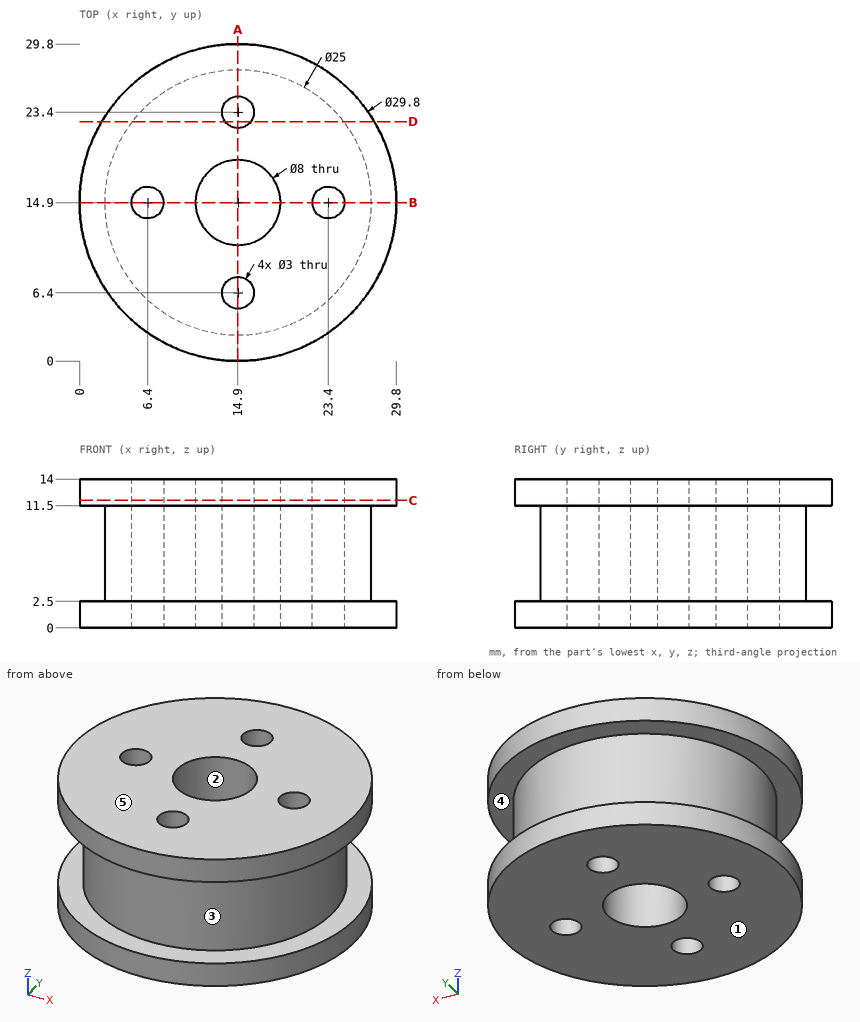
Geometry check sheet. Reference: drawing and pictorial views, mm from the part's lowest x, y, z. A direction names the side the tool comes from. Coordinates: 2 decimals unless noted, no trailing zeros. Order: outer loops, then holes, each group sorted by start corner. A loop starts at its lowest first (then second) coordinate and runs counter-clockwise, first axis right, second up. Notation, with made-up numbers: (-9, 70) - (18, 70) arc R20 cw to (18, 101) - close; hole circle Ø3 at (-20.75, -9.75). An arc over 180 degrees is marked (long way). One line per item, written item: value.
(1) Access from +Z, -Z, +X, -X, +Y, -Y to the whole of each face (thin tool, end or side, straight path). Record for the marked faces 4 and 5.
Data:
face 4: none
face 5: +Z, +X, -X, +Y, -Y
(2) Sectioned sample at A-A (x = 14.9). Enter the section's corners in (y, z).
Data:
outline: (0, 0) - (4.9, 0) - (4.9, 14) - (0, 14) - (0, 11.5) - (2.4, 11.5) - (2.4, 2.5) - (0, 2.5) - close; (7.9, 0) - (10.9, 0) - (10.9, 14) - (7.9, 14) - close; (18.9, 0) - (21.9, 0) - (21.9, 14) - (18.9, 14) - close; (24.9, 0) - (29.8, 0) - (29.8, 2.5) - (27.4, 2.5) - (27.4, 11.5) - (29.8, 11.5) - (29.8, 14) - (24.9, 14) - close
(3) Depth check by flat-ended pin: pin 1 Ø1 at (x, y) = (24.5, 22) entering from -Z; pin 2 Ø6 at (x, z) = (7, 2) entering from +Y; pin 3 Ø3 at (x, z) = (5.5, 10.5) entering from -Y; pin 4 Ø1 at (x, z) = (20.5, 9.5) entering from +Y. Enter the tip coordinate at first touch or a pass-through.
Data:
pin 1: stops at z = 0
pin 2: stops at y = 28.97
pin 3: stops at y = 2.51
pin 4: stops at y = 26.31
(4) Sectioned sample at D-D (y = 22.5). Enter the section's corners in (x, z), and give its area (3 significant figures).
Data:
outline: (2.08, 0) - (13.7, 0) - (13.7, 14) - (2.08, 14) - (2.08, 11.5) - (4.98, 11.5) - (4.98, 2.5) - (2.08, 2.5) - close; (16.1, 0) - (27.72, 0) - (27.72, 2.5) - (24.82, 2.5) - (24.82, 11.5) - (27.72, 11.5) - (27.72, 14) - (16.1, 14) - close
area: 273 mm^2
(5) Thickness scan on probe 1 along Y at (x, z) = (14.9, 8); probe 2 along Z at (x, y) = (26.75, 9.75); probe 3 along X at (y, z) = (12, 9.25) (3 decimals). Record the ranges inside material, lowest first. Write a range as from..to.
Data:
probe 1: y = 2.4..4.9, 7.9..10.9, 18.9..21.9, 24.9..27.4
probe 2: z = 0..2.5, 11.5..14
probe 3: x = 2.741..12.145, 17.655..27.059
(6) Sectioned sample at C-C (z = 12). Enter the section's corners in (x, y), and give its area (3 significant figures).
Data:
outline: circle Ø29.8 at (14.9, 14.9); hole circle Ø3 at (6.4, 14.9); hole circle Ø8 at (14.9, 14.9); hole circle Ø3 at (14.9, 6.4); hole circle Ø3 at (14.9, 23.4); hole circle Ø3 at (23.4, 14.9)
area: 619 mm^2
(7) Release check for a two-part mould opening along Z. For the marked faces 1, 2 and 3 record: +Z half, -Z half, draft (parallel to the pull), parting line (faces both ways), or undercut.
Data:
face 1: -Z half
face 2: draft
face 3: undercut
